The model under review builds one solid part; all positions refer to its coordinate system, in mm. A direction names the side the tool comes from. Give positions to 0.01 mm unless a question says otherwise; leave off trailing zeros. Write each loop counter-clockwise with the first axis right and the second up, starting at its lowest first coordinate (ties: lowest second). Pieces come first, ordered by that corner, then holes. Notation, with made-up numbers: (-38.75, -16) - (-32.75, -16) arc R18 cw to (-32.75, -5) - close; hole circle Ø6 at (70.25, 46.5). An arc over 180 degrees is marked (long way). Write item = value, one per line.
```python
from build123d import *
from build123d import SkipClean  # not in build123d's __all__

# Parameters (mm, degrees)
F1_DEPTH = 50.8
F2_DEPTH = 19.05
F3_DEPTH = 6.35
F4_DEPTH = 6.35


# Not quite as in the source:
# - after a boolean that leaves OpenCascade's solid faulty, fix() repairs it


with BuildPart() as f1:
    # F0 (on Top) → F1 (new body)
    with BuildSketch(Plane.XY):
        with BuildLine():
            Line((-7.3013131592, 69.4673543915), (-7.965068901, 75.7825684271))
            ThreePointArc((-7.965068901, 75.7825684271), (-76.0955705483, -3.9879998657), (0, -76.2))
            Line((0, -76.2), (0, -69.85))
            ThreePointArc((0, -69.85), (-69.7542730026, -3.6556665436), (-7.3013131592, 69.4673543915))
        make_face()
        with BuildLine():
            Line((0, 69.85), (0, 76.2))
            ThreePointArc((0, 76.2), (-3.9879998657, 76.0955705483), (-7.965068901, 75.7825684271))
            Line((-7.965068901, 75.7825684271), (-7.3013131592, 69.4673543915))
            ThreePointArc((-7.3013131592, 69.4673543915), (-3.6556665436, 69.7542730026), (0, 69.85))
        make_face()
        with BuildLine():
            ThreePointArc((0, -76.2), (3.9879998657, -76.0955705483), (7.965068901, -75.7825684271))
            Line((7.965068901, -75.7825684271), (7.3013131592, -69.4673543915))
            ThreePointArc((7.3013131592, -69.4673543915), (3.6556665436, -69.7542730026), (0, -69.85))
            Line((0, -69.85), (0, -76.2))
        make_face()
        with BuildLine():
            ThreePointArc((7.965068901, -75.7825684271), (56.6276357014, -50.9877522045), (76.2, 0))
            ThreePointArc((76.2, 0), (53.8815367264, 53.8815367264), (0, 76.2))
            Line((0, 76.2), (0, 69.85))
            ThreePointArc((0, 69.85), (49.3914086659, 49.3914086659), (69.85, 0))
            ThreePointArc((69.85, 0), (51.9086660596, -46.7387728542), (7.3013131592, -69.4673543915))
            Line((7.3013131592, -69.4673543915), (7.965068901, -75.7825684271))
        make_face()
    extrude(amount=F1_DEPTH)

    # F0 (on Top) → F2 (join)
    with BuildSketch(Plane.XY):
        with BuildLine():
            ThreePointArc((-7.965068901, 75.7825684271), (-3.9879998657, 76.0955705483), (0, 76.2))
            Line((0, 76.2), (0, 88.9))
            ThreePointArc((0, 88.9), (-4.65266651, 88.7781656397), (-9.2925803845, 88.4129964982))
            Line((-9.2925803845, 88.4129964982), (-7.965068901, 75.7825684271))
        make_face()
        with BuildLine():
            Line((9.2925803845, -88.4129964982), (7.965068901, -75.7825684271))
            ThreePointArc((7.965068901, -75.7825684271), (3.9879998657, -76.0955705483), (0, -76.2))
            Line((0, -76.2), (0, -88.9))
            ThreePointArc((0, -88.9), (4.65266651, -88.7781656397), (9.2925803845, -88.4129964982))
        make_face()
    extrude(amount=F2_DEPTH)

    # F0 (on Top) → F3 (cut)
    with BuildSketch(Plane.XY):
        with BuildLine():
            Line((9.2925803845, -88.4129964982), (7.965068901, -75.7825684271))
            ThreePointArc((7.965068901, -75.7825684271), (3.9879998657, -76.0955705483), (0, -76.2))
            Line((0, -76.2), (0, -88.9))
            ThreePointArc((0, -88.9), (4.65266651, -88.7781656397), (9.2925803845, -88.4129964982))
        make_face()
        with BuildLine():
            ThreePointArc((-7.965068901, 75.7825684271), (-3.9879998657, 76.0955705483), (0, 76.2))
            Line((0, 76.2), (0, 88.9))
            ThreePointArc((0, 88.9), (-4.65266651, 88.7781656397), (-9.2925803845, 88.4129964982))
            Line((-9.2925803845, 88.4129964982), (-7.965068901, 75.7825684271))
        make_face()
    with SkipClean():  # cleaning this boolean's faces spoils the solid; the shape is the same uncleaned
        extrude(amount=F3_DEPTH, mode=Mode.SUBTRACT)

    # F0 (on Top) → F4 (join)
    with BuildSketch(Plane.XY):
        with BuildLine():
            Line((0, 0), (-7.3013131592, 69.4673543915))
            ThreePointArc((-7.3013131592, 69.4673543915), (-69.7542730026, -3.6556665436), (0, -69.85))
            Line((0, -69.85), (0, 0))
        make_face()
        with BuildLine():
            Line((0, 0), (0, 69.85))
            ThreePointArc((0, 69.85), (-3.6556665436, 69.7542730026), (-7.3013131592, 69.4673543915))
            Line((-7.3013131592, 69.4673543915), (0, 0))
        make_face()
        with BuildLine():
            ThreePointArc((69.85, 0), (49.3914086659, 49.3914086659), (0, 69.85))
            Line((0, 69.85), (0, 0))
            Line((0, 0), (7.3013131592, -69.4673543915))
            ThreePointArc((7.3013131592, -69.4673543915), (51.9086660596, -46.7387728542), (69.85, 0))
        make_face()
        with BuildLine():
            ThreePointArc((0, -69.85), (3.6556665436, -69.7542730026), (7.3013131592, -69.4673543915))
            Line((7.3013131592, -69.4673543915), (0, 0))
            Line((0, 0), (0, -69.85))
        make_face()
    extrude(amount=F4_DEPTH)

    add(f1.part.fix(), mode=Mode.REPLACE)


solid = f1.part
```
1. Take a section at B-B on x = -27. Give the boundary of the cut face in (y, z).
Findings below:
outline = (-71.26, 0) - (71.26, 0) - (71.26, 50.8) - (64.42, 50.8) - (64.42, 6.35) - (-64.42, 6.35) - (-64.42, 50.8) - (-71.26, 50.8) - close
2. For line 1 (Y direction, x = -7.5, z = 24.5); line 2 (Z direction, x = 57, y = 8.5); line 3 (Y direction, x = -26, z = 37), list the stretches that pass through material, from the lowest coordinate up. Write a range as from..to.
Findings below:
line_1 = -75.83..-69.45, 69.45..75.83
line_2 = 0..6.35
line_3 = -71.63..-64.83, 64.83..71.63
3. Draft analysis for pull direction Y (two halves, no side actions). For faces 1 (the cylindrical face through (-4.59, 88.78, 12.61)), 2 (the flat face through (-8.64, 82.19, 12.61)), 3 (the cylindrical face through (4.59, -88.78, 12.61)), 4 (the flat face through (0, 82, 13)), state which applies: +Y half, -Y half, draft (parallel to the pull), parting line (faces both ways), or undercut.
Findings below:
face_1 = +Y half
face_2 = undercut
face_3 = -Y half
face_4 = draft
4. Take a section at C-C on y = 12. Give the boundary of the cut face in (x, z).
Findings below:
outline = (-75.25, 0) - (75.25, 0) - (75.25, 50.8) - (68.81, 50.8) - (68.81, 6.35) - (-68.81, 6.35) - (-68.81, 50.8) - (-75.25, 50.8) - close
5. Take a section at A-A on z = 26.5. Give the boundary of the cut face in (x, y), and give its area (3 significant figures).
Findings below:
outline = circle Ø152.4 at (0, 0); hole circle Ø139.7 at (0, 0)
area = 2,910 mm²
6. Machinability: for faces 5 (the flat face through (8.64, -82.19, 12.61)), 6 (the flat face through (-1, 1, 6.35)), 7 (the flat face through (0, -82, 13)), which of the approach directions +Z, -Z, +X, -X, +Y, -Y give a long, thin tool a straight path to every point of the face, cutting with its end or side? Answer none if there is none.
Findings below:
face_5 = +Z, -Z, +X
face_6 = +Z
face_7 = +Z, -Z, -X, -Y
7. Insertion check: P1, Ø12, axis at x = 5, z = 6.5, coming from the -Y side; P2, Ø10, axis at x = 4, y = -81.5, coming from the +Z side; P3, Ø3, axis at x = -17, z = 19.5, coming from the -Y side; P4, Ø4.5, axis at x = 2.5, y = -79, coming from the -Z side. Each pin has a flat end and moves straight along its axis. Give the tip position at first contact, or say it passes through.
Findings below:
P1 = -88.9
P2 = 19.05
P3 = -74.61
P4 = 6.35
